```python
from build123d import *

# Parameters (mm, degrees)
FSAE_CHASSIS_1_5_X_1_INCH_RECT_1_DEPTH = 40
CUT_EXTRUDE1_DEPTH                     = 52.069193258
CUT_EXTRUDE1_DEPTH_BACK                = 52.069193258
F_13_0_13_DIAMETER_HOLE2_D             = 13


with BuildPart() as part:
    # Sketch15 → Fsae chassis 1_5 X 1 INCH RECT(1) (new body)
    with BuildSketch(Plane(origin=(0, 0, 0), x_dir=(0, 0, -1), z_dir=(1, 0, 0))):
        with BuildLine():
            Line((-9.4488, 19.05), (9.4488, 19.05))
            ThreePointArc((9.4488, 19.05), (11.747745567, 18.097745567), (12.7, 15.7988))
            Line((12.7, 15.7988), (12.7, -15.7988))
            ThreePointArc((12.7, -15.7988), (11.747745567, -18.097745567), (9.4488, -19.05))
            Line((9.4488, -19.05), (-9.4488, -19.05))
            ThreePointArc((-9.4488, -19.05), (-11.747745567, -18.097745567), (-12.7, -15.7988))
            Line((-12.7, -15.7988), (-12.7, 15.7988))
            ThreePointArc((-12.7, 15.7988), (-11.747745567, 18.097745567), (-9.4488, 19.05))
        make_face()
        with BuildLine():
            Line((-9.4488, -17.399), (9.4488, -17.399))
            ThreePointArc((9.4488, -17.399), (10.580312271, -16.930312271), (11.049, -15.7988))
            Line((11.049, -15.7988), (11.049, 15.7988))
            ThreePointArc((11.049, 15.7988), (10.580312271, 16.930312271), (9.4488, 17.399))
            Line((9.4488, 17.399), (-9.4488, 17.399))
            ThreePointArc((-9.4488, 17.399), (-10.580312271, 16.930312271), (-11.049, 15.7988))
            Line((-11.049, 15.7988), (-11.049, -15.7988))
            ThreePointArc((-11.049, -15.7988), (-10.580312271, -16.930312271), (-9.4488, -17.399))
        make_face(mode=Mode.SUBTRACT)
    extrude(amount=FSAE_CHASSIS_1_5_X_1_INCH_RECT_1_DEPTH)

    # Sketch16 → Cut-Extrude1 (cut, two sides: drawn at the far end of the back side and taken through both)
    with BuildSketch(Plane(origin=(0, 0, -12.7), x_dir=(-1, 0, 0), z_dir=(0, 0, -1)).offset(-CUT_EXTRUDE1_DEPTH_BACK)):
        with BuildLine():
            Line((-15.88, 11), (-10.18, 11))
            ThreePointArc((-10.18, 11), (-4.903003105, 11.708724672), (0, 13.784669623))
            Line((0, 13.784669623), (0, -13.784669623))
            ThreePointArc((0, -13.784669623), (-4.903003105, -11.708724672), (-10.18, -11))
            Line((-10.18, -11), (-15.88, -11))
            ThreePointArc((-15.88, -11), (-26.88, 0), (-15.88, 11))
        make_face()
    extrude(amount=CUT_EXTRUDE1_DEPTH + CUT_EXTRUDE1_DEPTH_BACK, mode=Mode.SUBTRACT)

    # Ø13.0 (13) Diameter Hole2 (through all)
    with Locations(Plane(origin=(0, 19.05, 0), x_dir=(1, 0, 0), z_dir=(0, 1, 0))):
        with Locations((12, 0)):
            Hole(F_13_0_13_DIAMETER_HOLE2_D / 2)


solid = part.part
```
Work out the finished part from the listing and answer in its coordinate system (mm). A direction names the side the tool comes from. Round coordinates to 2 decimals unless told otherwise and drop trailing zeros. Write each loop counter-clockwise with the first axis right and the second up, starting at its lowest first coordinate (ties: lowest second). Pieces come first, ordered by that corner, then holes. Notation, with made-up numbers: (4, 28) -> (20, 28) arc R17 ccw to (20, 55) -> close; hole circle Ø7 at (29, -39). An arc over 180 degrees is marked (long way). Write each question's results on one line, items separated by ' | '.
1) Which of the six approach directions +Z, -Z, +X, -X, +Y, -Y give full straight-line access (tool end or side, diameter ignored) to faces 5 (the cylindrical face through (19.72, -16.94, -10.57)), 6 (the cylindrical face through (4.83, -11.73, -11.86)), 7 (the flat face through (20, -19.05, 0))?
Findings:
face 5: +X, -X | face 6: +Z, -Z, -X | face 7: +Z, -Z, +X, -X, -Y
2) The part is cut by section B-B (z = 0). Write down the section's boundary in (x, y).
Findings:
outline: (0, -19.05) -> (5.5, -19.05) -> (5.5, -17.4) -> (0, -17.4) -> close; (0, 17.4) -> (5.5, 17.4) -> (5.5, 19.05) -> (0, 19.05) -> close; (18.5, -19.05) -> (40, -19.05) -> (40, -17.4) -> (18.5, -17.4) -> close; (18.5, 17.4) -> (40, 17.4) -> (40, 19.05) -> (18.5, 19.05) -> close
3) Flat-ended cylindrical pins translate along their axes: pin 1 (1.8 mm diameter, centred on x = 13, z = 12, fed in from +Y); pin 2 (6 mm diameter, centred on y = -12.5, z = 6.5, fed in from -X); pin 3 (1.8 mm diameter, centred on x = 14, z = -11.5, fed in from -Y); pin 4 (1.3 mm diameter, centred on x = 13.5, z = -12, fed in from +Y). Find the tip coordinate at first contact, or state that the pin passes through.
Findings:
pin 1: stops at y = 18.6 | pin 2: passes through | pin 3: stops at y = -18.84 | pin 4: stops at y = 18.44
4) The part is cut by section A-A (x = 12). State how many separate pieces and enclosed holes the cut face has, and give its area (3 significant figures).
Findings:
separate pieces: 4 | enclosed holes: 0 | area: 76.3 mm²
5) Consider line 1 along Y through (x, z) = (37, -0.5); line 2 along Z through (x, y) = (36, 14.5). Determine where each line is inside the solid, lowest interval first. Write a range as [from, to].
Findings:
line 1: y = [-19.05, -17.4], [17.4, 19.05] | line 2: z = [-12.7, -11.05], [11.05, 12.7]
6) The part is cut by section C-C (y = 0). Write down the section's boundary in (x, z), and give its area (3 significant figures).
Findings:
outline: (26.88, -12.7) -> (40, -12.7) -> (40, -11.05) -> (26.88, -11.05) -> close; (26.88, 11.05) -> (40, 11.05) -> (40, 12.7) -> (26.88, 12.7) -> close | area: 43.3 mm²
7) For a pull along X with two mould halves and no side action, classify faces 1 (the flat face through (40, 0.1, -11.3)), 2 (the cylindrical face through (5.8, -18.24, -1.95)), 3 (the cylindrical face through (19.72, 16.94, 10.57)), 4 (the cylindrical face through (26.877, -0.242, 11.886)) as +X half, -X half, draft (parallel to the pull), parting line (faces both ways), or undercut.
Findings:
face 1: +X half | face 2: undercut | face 3: draft | face 4: -X half
8) The part is cut by section D-D (x = 35.5). Write down the section's boundary in (y, z), and give its area (3 significant figures).
Findings:
outline: (-19.05, -9.45) arc R3.25 ccw to (-15.8, -12.7) -> (15.8, -12.7) arc R3.25 ccw to (19.05, -9.45) -> (19.05, 9.45) arc R3.25 ccw to (15.8, 12.7) -> (-15.8, 12.7) arc R3.25 ccw to (-19.05, 9.45) -> close; hole (-17.4, -9.45) arc R1.6 ccw to (-15.8, -11.05) -> (15.8, -11.05) arc R1.6 ccw to (17.4, -9.45) -> (17.4, 9.45) arc R1.6 ccw to (15.8, 11.05) -> (-15.8, 11.05) arc R1.6 ccw to (-17.4, 9.45) -> close | area: 192 mm²
